```python
from build123d import *
from OCP.BRepFilletAPI import BRepFilletAPI_MakeChamfer

# Parameters (mm, degrees)
ESBO_O1_W                  = 47.75
ESBO_O1_H                  = 28.75
RESSALTO_EXTRUS_O1_DEPTH   = 17.53
ESBO_O3_W                  = 55.113346814
ESBO_O3_H                  = 32.23245858
ESBO_O3_W_2                = 45.28
ESBO_O3_H_2                = 25.85
CORTE_EXTRUS_O1_DEPTH      = 15.22
CORTE_EXTRUS_O2_DEPTH      = 17
CORTE_EXTRUS_O2_DEPTH_BACK = 33.22
ESBO_O4_W                  = 35.95
ESBO_O4_H                  = 18.14
ESBO_O5_W                  = 41.28
ESBO_O5_H                  = 21.85
CORTE_EXTRUS_O3_DEPTH      = 15.22
CHANFRO1_SIZE              = 1
CHANFRO1_SIZE2             = 2.144506921
CHANFRO2_SIZE              = 1
CHANFRO2_SIZE2             = 2.144506921
CHANFRO3_SIZE              = 1
CHANFRO3_SIZE2             = 1.539864964
FILETE1_R                  = 1.5
CORTE_EXTRUS_O4_DEPTH      = 15
CORTE_EXTRUS_O4_DEPTH_BACK = 44.22
CORTE_EXTRUS_O5_DEPTH      = 0.4
ESBO_O8_W                  = 24.82
ESBO_O8_H                  = 1
CORTE_EXTRUS_O6_DEPTH      = 0.4
ESBO_O9_W                  = 9
ESBO_O9_H                  = 6.324480946
RESSALTO_EXTRUS_O2_DEPTH   = 1.45
ESBO_O10_W                 = 9
ESBO_O10_H                 = 6.324480946
RESSALTO_EXTRUS_O3_DEPTH   = 1.45
ESBO_O11_W                 = 9
ESBO_O11_H                 = 6.324480946
RESSALTO_EXTRUS_O4_DEPTH   = 1.45
CHANFRO4_SIZE              = 3
CHANFRO4_SIZE2             = 3.575260778


with BuildPart() as part:
    # Esboço1 → Ressalto-extrusão1 (new body)
    with BuildSketch(Plane.XY):
        Rectangle(ESBO_O1_W, ESBO_O1_H)
    extrude(amount=RESSALTO_EXTRUS_O1_DEPTH)

    # Esboço3 → Corte-extrusão1 (cut)
    with BuildSketch(Plane(origin=(0, 0, 0), x_dir=(-1, 0, 0), z_dir=(0, 0, -1))):
        Rectangle(ESBO_O3_W, ESBO_O3_H)
        Rectangle(ESBO_O3_W_2, ESBO_O3_H_2, mode=Mode.SUBTRACT)
    extrude(amount=-CORTE_EXTRUS_O1_DEPTH, mode=Mode.SUBTRACT)

    # Esboço4 → Corte-extrusão2 (cut, two sides: drawn at the far end of the back side and taken through both)
    with BuildSketch(Plane.XY.offset(17.53).offset(-CORTE_EXTRUS_O2_DEPTH_BACK)):
        Rectangle(ESBO_O4_W, ESBO_O4_H)
    extrude(amount=CORTE_EXTRUS_O2_DEPTH + CORTE_EXTRUS_O2_DEPTH_BACK, mode=Mode.SUBTRACT)

    # Esboço5 → Corte-extrusão3 (cut)
    with BuildSketch(Plane(origin=(0, 0, 0), x_dir=(-1, 0, 0), z_dir=(0, 0, -1))):
        Rectangle(ESBO_O5_W, ESBO_O5_H)
    extrude(amount=-CORTE_EXTRUS_O3_DEPTH, mode=Mode.SUBTRACT)

    # Chanfro1
    chanfro1_edges = [part.edges().sort_by_distance(p)[0] for p in [
        (17.975, 0, 17.53),
    ]]
    chanfro1_side = [part.faces().sort_by_distance(p)[0] for p in [
        (17.975, 0, 16.375),
    ]]
    chamfer(chanfro1_edges, length=CHANFRO1_SIZE, length2=CHANFRO1_SIZE2, reference=chanfro1_side[0])

    # Chanfro2
    chanfro2_edges = [part.edges().sort_by_distance(p)[0] for p in [
        (-17.975, 0, 17.53),
    ]]
    chanfro2_side = [part.faces().sort_by_distance(p)[0] for p in [
        (-17.975, 0, 16.375),
    ]]
    chamfer(chanfro2_edges, length=CHANFRO2_SIZE, length2=CHANFRO2_SIZE2, reference=chanfro2_side[0])

    # Chanfro3: one chamfer whose edges measure the first distance from different faces: ONE call of the kernel's chamfer builder (chamfer() names one face for all edges)
    chanfro3_edges_1 = [part.edges().sort_by_distance(p)[0] for p in [
        (0, -9.07, 17.53),
    ]]
    chanfro3_side_1 = [part.faces().sort_by_distance(p)[0] for p in [
        (0, -9.07, 16.39568424),
    ]]
    chanfro3_edges_2 = [part.edges().sort_by_distance(p)[0] for p in [
        (0, 9.07, 17.53),
    ]]
    chanfro3_side_2 = [part.faces().sort_by_distance(p)[0] for p in [
        (0, 9.07, 16.39568424),
    ]]
    chanfro3 = BRepFilletAPI_MakeChamfer(part.part.solid().wrapped)
    for e in chanfro3_edges_1:
        chanfro3.Add(CHANFRO3_SIZE, CHANFRO3_SIZE2, e.wrapped, chanfro3_side_1[0].wrapped)  # the first distance lies on this face
    for e in chanfro3_edges_2:
        chanfro3.Add(CHANFRO3_SIZE, CHANFRO3_SIZE2, e.wrapped, chanfro3_side_2[0].wrapped)  # the first distance lies on this face
    add(Compound.cast(chanfro3.Shape()), mode=Mode.REPLACE)

    # Filete1
    filete1_edges = [part.edges().sort_by_distance(p)[0] for p in [
        (23.875, 0, 17.53),
        (0, 14.375, 17.53),
        (-23.875, 0, 17.53),
        (0, -14.375, 17.53),
    ]]
    fillet(filete1_edges, radius=FILETE1_R)

    # Esboço6 → Corte-extrusão4 (cut, two sides: drawn at the far end of the back side and taken through both)
    with BuildSketch(Plane(origin=(0, 12.925, 0), x_dir=(1, 0, 0), z_dir=(0, 1, 0)).offset(-CORTE_EXTRUS_O4_DEPTH_BACK)):
        Polygon((-11.41, -7.895519054), (-11.41, -7.22), (-12.41, -7.22), (-12.41, -15.22), (12.41, -15.22), (12.41, -7.22), (11.41, -7.22), (11.41, -7.895519054), (11.41, -14.544480946), (2.41, -14.544480946), (2.41, -7.22), (-2.41, -7.22), (-2.41, -14.544480946), (-11.41, -14.544480946), align=None)
    extrude(amount=CORTE_EXTRUS_O4_DEPTH + CORTE_EXTRUS_O4_DEPTH_BACK, mode=Mode.SUBTRACT)

    # Esboço7 → Corte-extrusão5 (cut)
    with BuildSketch(Plane(origin=(0, 12.925, 0), x_dir=(1, 0, 0), z_dir=(0, 1, 0))):
        Polygon((-12.410087555, -8.22), (12.410087555, -8.22), (12.41, -7.22), (-12.41, -7.22), align=None)
    extrude(amount=-CORTE_EXTRUS_O5_DEPTH, mode=Mode.SUBTRACT)

    # Esboço8 → Corte-extrusão6 (cut)
    with BuildSketch(Plane.XZ.offset(12.925)):
        with Locations((0, 7.72)):
            Rectangle(ESBO_O8_W, ESBO_O8_H)
    extrude(amount=-CORTE_EXTRUS_O6_DEPTH, mode=Mode.SUBTRACT)

    # Esboço9 → Ressalto-extrusão2 (add)
    with BuildSketch(Plane(origin=(0, 12.925, 0), x_dir=(1, 0, 0), z_dir=(0, 1, 0))):
        with Locations((-6.91, -11.382240473)):
            Rectangle(ESBO_O9_W, ESBO_O9_H)
    extrude(amount=RESSALTO_EXTRUS_O2_DEPTH)

    # Esboço10 → Ressalto-extrusão3 (add)
    with BuildSketch(Plane(origin=(0, 12.925, 0), x_dir=(1, 0, 0), z_dir=(0, 1, 0))):
        with Locations((6.91, -11.382240473)):
            Rectangle(ESBO_O10_W, ESBO_O10_H)
    extrude(amount=RESSALTO_EXTRUS_O3_DEPTH)

    # Esboço11 → Ressalto-extrusão4 (add)
    with BuildSketch(Plane.XZ.offset(12.925)):
        with Locations((6.91, 11.382240473)):
            Rectangle(ESBO_O11_W, ESBO_O11_H)
        Polygon((-2.41, 8.22), (-2.41, 14.544480946), (-6.91, 14.544480946), (-11.41, 14.544480946), (-11.41, 8.22), align=None)
    extrude(amount=RESSALTO_EXTRUS_O4_DEPTH)

    # Chanfro4: one chamfer whose edges measure the first distance from different faces: ONE call of the kernel's chamfer builder (chamfer() names one face for all edges)
    chanfro4_edges_1 = [part.edges().sort_by_distance(p)[0] for p in [
        (-6.91, 14.375, 14.544480946),
    ]]
    chanfro4_side_1 = [part.faces().sort_by_distance(p)[0] for p in [
        (-6.91, 12.65, 14.544480946),
    ]]
    chanfro4_edges_2 = [part.edges().sort_by_distance(p)[0] for p in [
        (6.91, 14.375, 14.544480946),
    ]]
    chanfro4_side_2 = [part.faces().sort_by_distance(p)[0] for p in [
        (6.91, 12.65, 14.544480946),
    ]]
    chanfro4_edges_3 = [part.edges().sort_by_distance(p)[0] for p in [
        (6.91, -14.375, 14.544480946),
    ]]
    chanfro4_side_3 = [part.faces().sort_by_distance(p)[0] for p in [
        (6.91, -12.65, 14.544480946),
    ]]
    chanfro4_edges_4 = [part.edges().sort_by_distance(p)[0] for p in [
        (-6.91, -14.375, 14.544480946),
    ]]
    chanfro4_side_4 = [part.faces().sort_by_distance(p)[0] for p in [
        (-6.91, -12.65, 14.544480946),
    ]]
    chanfro4 = BRepFilletAPI_MakeChamfer(part.part.solid().wrapped)
    for e in chanfro4_edges_1:
        chanfro4.Add(CHANFRO4_SIZE, CHANFRO4_SIZE2, e.wrapped, chanfro4_side_1[0].wrapped)  # the first distance lies on this face
    for e in chanfro4_edges_2:
        chanfro4.Add(CHANFRO4_SIZE, CHANFRO4_SIZE2, e.wrapped, chanfro4_side_2[0].wrapped)  # the first distance lies on this face
    for e in chanfro4_edges_3:
        chanfro4.Add(CHANFRO4_SIZE, CHANFRO4_SIZE2, e.wrapped, chanfro4_side_3[0].wrapped)  # the first distance lies on this face
    for e in chanfro4_edges_4:
        chanfro4.Add(CHANFRO4_SIZE, CHANFRO4_SIZE2, e.wrapped, chanfro4_side_4[0].wrapped)  # the first distance lies on this face
    add(Compound.cast(chanfro4.Shape()), mode=Mode.REPLACE)

    # Chanfro5
    # the kernel refuses this chamfer: 2.383507185, 2 mm, written as the material it takes off along each edge
    with BuildSketch(Plane(origin=(-11.41, 14.375, 8.22), x_dir=(0, 0.024939322090234445, 0.9996889667359941), z_dir=(1, 0, 0))) as chanfro5_piece_1_section:
        with BuildLine():
            Line((2.457306387, 0), (-0.124419196, 2.058820987))
            Line((-0.124419196, 2.058820987), (-0.172074512, 2.057632126))
            ThreePointArc((-0.172074512, 2.057632126), (-0.073358824, 1.029132353), (-0.047655317, -0.001188861))
            Line((-0.047655317, -0.001188861), (0.001188861, -0.047655317))
            ThreePointArc((0.001188861, -0.047655317), (1.229077869, -0.01702307), (2.458495248, -0.047655317))
            Line((2.458495248, -0.047655317), (2.457306387, 0))
        make_face()
    chanfro5_piece_1 = extrude(amount=9, mode=Mode.PRIVATE)
    chanfro5_piece_1 = split(chanfro5_piece_1, bisect_by=Plane(origin=(-6.91, 12.525, 9.020332746), z_dir=(0, 1, 0)), keep=Keep.TOP, mode=Mode.PRIVATE)
    add(chanfro5_piece_1, mode=Mode.SUBTRACT)
    with BuildSketch(Plane(origin=(11.41, 14.375, 8.22), x_dir=(0, 0.024939322090234445, 0.9996889667359941), z_dir=(-1, 0, 0))) as chanfro5_piece_2_section:
        with BuildLine():
            Line((2.457306387, 0), (-0.124419196, -2.058820987))
            Line((-0.124419196, -2.058820987), (-0.172074512, -2.057632126))
            ThreePointArc((-0.172074512, -2.057632126), (-0.073358824, -1.029132353), (-0.047655317, 0.001188861))
            Line((-0.047655317, 0.001188861), (0.001188861, 0.047655317))
            ThreePointArc((0.001188861, 0.047655317), (1.229077869, 0.01702307), (2.458495248, 0.047655317))
            Line((2.458495248, 0.047655317), (2.457306387, 0))
        make_face()
    chanfro5_piece_2 = extrude(amount=9, mode=Mode.PRIVATE)
    chanfro5_piece_2 = split(chanfro5_piece_2, bisect_by=Plane(origin=(6.91, 12.525, 9.020332746), z_dir=(0, 1, 0)), keep=Keep.TOP, mode=Mode.PRIVATE)
    add(chanfro5_piece_2, mode=Mode.SUBTRACT)
    with BuildSketch(Plane(origin=(2.41, -14.375, 8.22), x_dir=(0, -0.024939322090234445, 0.9996889667359941), z_dir=(1, 0, 0))) as chanfro5_piece_3_section:
        with BuildLine():
            Line((2.457306387, 0), (-0.124419196, -2.058820987))
            Line((-0.124419196, -2.058820987), (-0.172074512, -2.057632126))
            ThreePointArc((-0.172074512, -2.057632126), (-0.073358824, -1.029132353), (-0.047655317, 0.001188861))
            Line((-0.047655317, 0.001188861), (0.001188861, 0.047655317))
            ThreePointArc((0.001188861, 0.047655317), (1.229077869, 0.01702307), (2.458495248, 0.047655317))
            Line((2.458495248, 0.047655317), (2.457306387, 0))
        make_face()
    chanfro5_piece_3 = extrude(amount=9, mode=Mode.PRIVATE)
    chanfro5_piece_3 = split(chanfro5_piece_3, bisect_by=Plane(origin=(6.91, -12.525, 9.020332746), z_dir=(0, -1, 0)), keep=Keep.TOP, mode=Mode.PRIVATE)
    add(chanfro5_piece_3, mode=Mode.SUBTRACT)
    with BuildSketch(Plane(origin=(-11.41, -14.375, 8.22), x_dir=(0, -0.03540953691366296, 0.9993728857116145), z_dir=(1, 0, 0))) as chanfro5_piece_4_section:
        with BuildLine():
            Line((2.062577027, 0), (-0.148230141, -2.452831528))
            Line((-0.148230141, -2.452831528), (-0.19587039, -2.45114355))
            ThreePointArc((-0.19587039, -2.45114355), (-0.091132758, -1.225812797), (-0.047640249, 0.001687978))
            Line((-0.047640249, 0.001687978), (0.001687978, 0.047640249))
            ThreePointArc((0.001687978, 0.047640249), (1.031683425, 0.011145701), (2.064265005, 0.047640249))
            Line((2.064265005, 0.047640249), (2.062577027, 0))
        make_face()
    chanfro5_piece_4 = extrude(amount=9, mode=Mode.PRIVATE)
    chanfro5_piece_4 = split(chanfro5_piece_4, bisect_by=Plane(origin=(-6.91, -12.525, 8.913974099), z_dir=(0, -1, 0)), keep=Keep.TOP, mode=Mode.PRIVATE)
    add(chanfro5_piece_4, mode=Mode.SUBTRACT)


solid = part.part
```
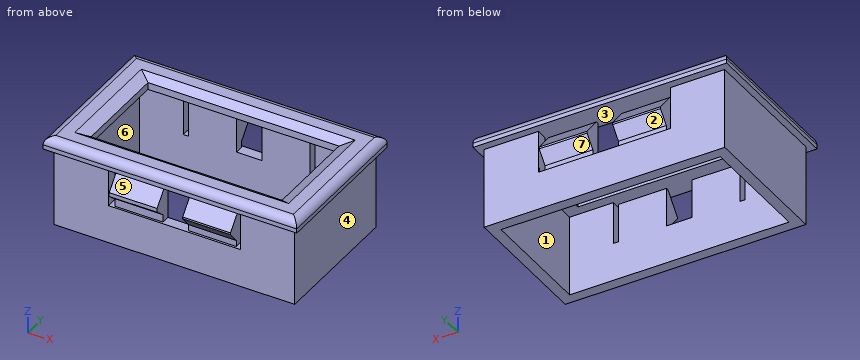
Check sheet for the modelled part. Datum: model origin and axes. Units: mm. Face numbers are marked on the shaded views. A direction names the side the tool comes from. Give positions to 0.01 mm unless a question says otherwise; leave off trailing zeros. Loops run counter-clockwise (first coordinate to the right, second up) from the corner with the lowest first, then second, coordinate; pieces in that order, holes last. Notation, with made-up numbers: (31, -18.75) - (53, -18.75) arc R11 cw to (53, -2.75) - close; hole circle Ø3 at (-4, 24). An arc over 180 degrees is marked (long way). One line per question, with ' | ' between items. Start each with the question number.
1. Cross-section at C-C, the plane y = 0.5. Enter the section's corners in (x, z) (1 decimal), plus the area to 3 significant figures.
2. Material ranges on line 1 along X through (y, z) = (-12, 9.75); line 2 along Y through (x, z) = (-14.5, 12.25) (3 decimals); line 3 along X through (y, z) = (-4.5, 14.75), recorded low to high. Write a range as [from, to].
3. Gauge pin test, flat ends, axial feed: pin 1 Ø6 at (x, z) = (5.5, 3.5) entering from -Y (3 decimals); pin 2 Ø4 at (y, z) = (13.5, 9.5) entering from -X; pin 3 Ø1 at (y, z) = (-13, 12.5) entering from +X. Record the tip position at first contact, or that the pin passes through.
4. Cross-section at D-D, the plane z = 13.5. Give the number of separate pieces and of enclosed holes in the cut face, plus the area to 3 significant figures.
5. Draft check along Z on the marked faces 6 and 7. Enter one of: released by +Z, released by -Z, zero draft, split by the parting line, or undercut.
6. Cross-section at A-A, the plane x = -1.5. Enter the section's corners in (y, z) (3 decimals).
7. Set-up check for the marked faces 1, 2, 3, 4 and 5: record each of +Z, -Z, +X, -X, +Y, -Y from which the full face is reachable in a straight line by a thin tool's end or side.
8. Cross-section at B-B, the plane x = 15.5. Enter the section's corners in (y, z) (3 decimals).
Check result:
1) outline: (-23.9, 15.2) - (-22.6, 15.2) - (-22.6, 0) - (-20.6, 0) - (-20.6, 15.2) - (-18, 15.2) - (-18, 16.5) - (-20.1, 17.5) - (-22.4, 17.5) arc R1.5 ccw to (-23.9, 16) - close; (18, 15.2) - (20.6, 15.2) - (20.6, 0) - (22.6, 0) - (22.6, 15.2) - (23.9, 15.2) - (23.9, 16) arc R1.5 ccw to (22.4, 17.5) - (20.1, 17.5) - (18, 16.5) - close | area: 85.0 mm2
2) line 1: x = [-22.64, -12.41], [-11.41, -2.41], [2.41, 11.41], [12.41, 22.64] | line 2: y = [-12.925, -10.925], [10.925, 12.925] | line 3: x = [-22.64, -20.64], [20.64, 22.64]
3) pin 1: stops at y = -12.925 | pin 2: stops at x = -22.64 | pin 3: stops at x = 22.64
4) separate pieces: 6 | enclosed holes: 0 | area: 217 mm2
5) face 6: zero draft | face 7: undercut
6) outline: (-14.375, 15.22) - (-9.07, 15.22) - (-9.07, 16.53) - (-10.61, 17.53) - (-12.875, 17.53) arc R1.5 ccw to (-14.375, 16.03) - close; (-12.925, 0) - (-10.925, 0) - (-10.925, 7.22) - (-12.925, 7.22) - close; (9.07, 15.22) - (14.375, 15.22) - (14.375, 16.03) arc R1.5 ccw to (12.875, 17.53) - (10.61, 17.53) - (9.07, 16.53) - close; (10.925, 0) - (12.925, 0) - (12.925, 7.22) - (10.925, 7.22) - close
7) face 1: -Z | face 2: +Y | face 3: none | face 4: -Z, +X, +Y, -Y | face 5: -Y
8) outline: (-14.375, 15.22) - (-12.925, 15.22) - (-12.925, 0) - (-10.925, 0) - (-10.925, 15.22) - (-9.07, 15.22) - (-9.07, 16.53) - (-10.61, 17.53) - (-12.875, 17.53) arc R1.5 ccw to (-14.375, 16.03) - close; (9.07, 15.22) - (10.925, 15.22) - (10.925, 0) - (12.925, 0) - (12.925, 15.22) - (14.375, 15.22) - (14.375, 16.03) arc R1.5 ccw to (12.875, 17.53) - (10.61, 17.53) - (9.07, 16.53) - close
